Part model, mm, in its own coordinate system. A direction names the side the tool comes from. Coordinates: 2 decimals unless noted, no trailing zeros. Loops run counter-clockwise (first coordinate to the right, second up) from the corner with the lowest first, then second, coordinate; pieces in that order, holes last. Notation, with made-up numbers: M 50.25,9.5 L 102.25,9.5 A19 ccw 102.25,34.5 Z; hole C 78.25,-21.75 d6. An arc over 180 degrees is marked long. Answer as a JSON object with one key per item and string values. Group by question number.
1. Saw through at D-D on y = 14. Write the cut outline in (x, z).
2. Saw through at B-B on x = -77.5. Write the cut outline in (y, z) (3 decimals), then the cut area to 3 significant figures.
3. 3-axis set-ups, long thin cutter, end or side, ignore diameter. For faces 1 (the face through (-78, 16, 0)), 2 (the face through (-76.3, 23.495, 20.1)): which of +Z, -Z, +X, -X, +Y, -Y reach the whole face in a straight line?
4. Saw through at A-A on y = 20. Write the cut outline in (x, z), then the cut area to 3 significant figures.
5. Drop flat-ended pins along their axis: pin 1 Ø4 at (x, y) = (-67, 15.5) entering from +Z; pin 2 Ø3 at (x, z) = (-67.5, 18) entering from +Y; pin 3 Ø5 at (y, z) = (13.5, 13.5) entering from +X. Give the stop position or say it passes through.
6. Drill centre lines: L1, parallel to Y at x = -73.25, z = 32 (3 decimals); L2, parallel to Z at x = -69.5, y = 24; L3, parallel to Z at x = -70.25, y = 14. Where is each one in solid material? Low to high.
7. Mould opens along Y. For faces 3 (the face through (-75, 31.75, 20)), 4 (the face through (-76.3, 8.255, 20.1)), 5 (the face through (-67.251, 16.097, 38.827)), 6 (the face through (-74, 0, 20)) say: released by +Y, released by -Y, zero draft, split by the parting line, or undercut.
8. Saw through at C-C on z = 35. Write the cut outline in (x, y) (3 decimals), then the cut area to 3 significant figures.
from build123d import *

# Parameters (mm, degrees)
REVOLVE1_ANGLE      = 30
SKETCH2_R           = 9.85774
BOSS_EXTRUDE1_DEPTH = 2.54
SKETCH3_R           = 9.85774
BOSS_EXTRUDE2_DEPTH = 12.7
SKETCH4_W           = 69.85
SKETCH4_H           = 31.75
CUT_REVOLVE1_ANGLE  = 30


with BuildPart() as part:
    # Sketch1 → Revolve1 (revolve)
    with BuildSketch(Plane.XY):
        Polygon((-80.01, 0), (-80.01, 8.255), (-78.74, 8.255), (-78.74, 23.495), (-80.01, 23.495), (-80.01, 31.75), (-76.2, 31.75), (-76.2, 0), align=None)
    revolve(axis=Axis((0, 0, 0), (0, 1, 0)), revolution_arc=REVOLVE1_ANGLE)

    # Sketch2 → Boss-Extrude1 (add)
    with BuildSketch(Plane(origin=(-71.095567884, 0, 19.05), x_dir=(0.258819045, 0, 0.965925826), z_dir=(-0.965925826, 0, 0.258819045))):
        with Locations((0, 15.875)):
            Circle(SKETCH2_R)
    extrude(amount=BOSS_EXTRUDE1_DEPTH)

    # Sketch3 → Boss-Extrude2 (add)
    with BuildSketch(Plane(origin=(-71.095567884, 0, 19.05), x_dir=(-0.258819045, 0, -0.965925826), z_dir=(0.965925826, 0, -0.258819045))):
        with Locations((0, 15.875)):
            Circle(SKETCH3_R)
    extrude(amount=BOSS_EXTRUDE2_DEPTH)

    # Sketch4 → Cut-Revolve1 (revolve, cut)
    with BuildSketch(Plane.XY):
        with Locations((-34.925, 15.875)):
            Rectangle(SKETCH4_W, SKETCH4_H)
    revolve(axis=Axis((0, 0, 0), (0, 1, 0)), revolution_arc=CUT_REVOLVE1_ANGLE, mode=Mode.SUBTRACT)


solid = part.part
Outcome:
{
 "1": {"outline": "M -78.74,0 L -76.2,0 A76.2 cw -75.51,10.21 L -69.32,8.56 A69.85 cw -64.31,27.25 L -70.5,28.91 A76.2 cw -65.99,38.1 L -68.19,39.37 A78.74 ccw Z; hole M -74.31,16.87 L -72.79,22.54 A76.2 ccw Z"},
 "2": {"outline": "M 0,0 L 31.75,0 L 31.75,19.883 L 23.495,19.883 L 23.495,13.919 L 8.255,13.919 L 8.255,19.883 L 0,19.883 Z", "area": "540 mm²"},
 "3": {"face 1": "-Z, +X, -X, +Y, -Y", "face 2": "+Z, -X"},
 "4": {"outline": "M -78.74,0 L -76.2,0 A76.2 cw -75.41,10.94 L -69.23,9.28 A69.85 cw -64.6,26.58 L -70.78,28.23 A76.2 cw -65.99,38.1 L -68.19,39.37 A78.74 ccw Z; hole M -74.31,16.87 L -72.79,22.54 A76.2 ccw Z", "area": "217 mm²"},
 "5": {"pin 1": "stops at z = 39.37", "pin 2": "stops at y = 25.73", "pin 3": "stops at x = -67.99"},
 "6": {"L1": "y = 0 to 8.255, 23.495 to 31.75", "L2": "z = 12.84 to 24.4, 31.24 to 39.64", "L3": "z = 8.8 to 28.84, 29.52 to 35.57"},
 "7": {"face 3": "released by +Y", "face 4": "undercut", "face 5": "zero draft", "face 6": "released by -Y"},
 "8": {"outline": "M -71.949,0 L -67.686,0 L -67.686,31.75 L -71.949,31.75 L -71.949,23.495 L -70.534,23.495 L -70.534,8.255 L -71.949,8.255 Z", "area": "114 mm²"}
}
